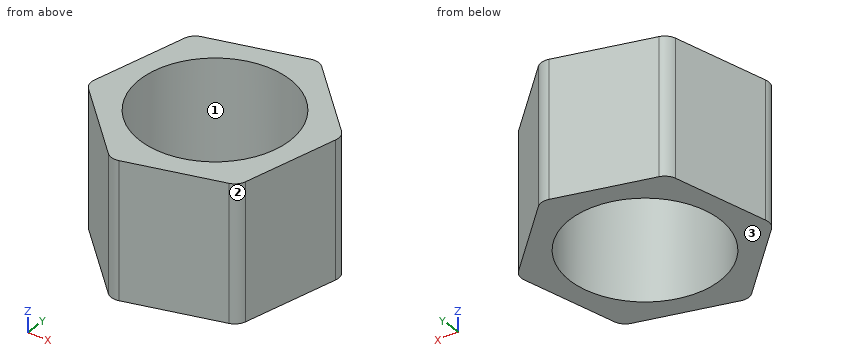
from build123d import *

# Parameters (mm, degrees)
SKETCH3_R           = 11
BOSS_EXTRUDE1_DEPTH = 20
FILLET1_R           = 2


with BuildPart() as part:
    # Sketch3 → Boss-Extrude1 (new body)
    with BuildSketch(Plane.XY):
        Polygon((11.666242226, -11.190716048), (15.524565497, 4.50790411), (3.858323271, 15.698620158), (-11.666242226, 11.190716048), (-15.524565497, -4.50790411), (-3.858323271, -15.698620158), align=None)
        Circle(SKETCH3_R, mode=Mode.SUBTRACT)
    extrude(amount=BOSS_EXTRUDE1_DEPTH)

    # Fillet1
    fillet1_edges = [part.edges().sort_by_distance(p)[0] for p in [
        (-3.858323271, -15.698620158, 10),
        (-15.524565497, -4.50790411, 10),
        (-11.666242226, 11.190716048, 10),
        (3.858323271, 15.698620158, 10),
        (15.524565497, 4.50790411, 10),
        (11.666242226, -11.190716048, 10),
    ]]
    fillet(fillet1_edges, radius=FILLET1_R)


solid = part.part
The listing builds one solid part. Answer for the finished solid, in the listing's coordinates (mm). Face numbers are marked on the shaded views. Give positions to 0.01 mm unless a question says otherwise; leave off trailing zeros. Loops run counter-clockwise (first coordinate to the right, second up) from the corner with the lowest first, then second, coordinate; pieces in that order, holes last. Notation, with made-up numbers: (64, -21) - (121, -21) arc R24 cw to (121, 1) - close; hole circle Ø7 at (64, 22.5). An arc over 180 degrees is marked (long way). Answer as a JSON object with one key per item and string values.
1. A cutting plane is placed at C-C (x = -8). Write down the section's boundary in (y, z), then the cut area to 3 significant figures.
Determined:
{"outline": "(-11.73, 0) - (-7.55, 0) - (-7.55, 20) - (-11.73, 20) - close; (7.55, 0) - (12.26, 0) - (12.26, 20) - (7.55, 20) - close", "area": "178 mm²"}
2. A cutting plane is placed at B-B (y = 0). Write down the section's boundary in (x, z).
Determined:
{"outline": "(-14.42, 0) - (-11, 0) - (-11, 20) - (-14.42, 20) - close; (11, 0) - (14.42, 0) - (14.42, 20) - (11, 20) - close"}
3. For a pull along Y with two mould halves and no side action, classify the marked faces 1, 2 and 3 as pulls with the +Y half, pulls with the -Y half, needs draft (parallel to the pull), parting line crosses it, or undercut.
Determined:
{"face 1": "undercut", "face 2": "pulls with the -Y half", "face 3": "needs draft"}
4. A cutting plane is placed at D-D (y = 13). Write down the section's boundary in (x, z), then the cut area to 3 significant figures.
Determined:
{"outline": "(-5.44, 0) - (6.67, 0) - (6.67, 20) - (-5.44, 20) - close", "area": "242 mm²"}
5. A cutting plane is placed at A-A (z = 2.25). Write down the section's boundary in (x, y), then the cut area to 3 significant figures.
Determined:
{"outline": "(-15.25, -3.39) arc R2 ccw to (-14.69, -5.31) - (-4.69, -14.9) arc R2 ccw to (-2.75, -15.38) - (10.56, -11.51) arc R2 ccw to (11.94, -10.07) - (15.25, 3.39) arc R2 ccw to (14.69, 5.31) - (4.69, 14.9) arc R2 ccw to (2.75, 15.38) - (-10.56, 11.51) arc R2 ccw to (-11.94, 10.07) - close; hole circle Ø22 at (0, 0)", "area": "298 mm²"}
6. Find the intervals of material crossed by L1, parallel to Y at x = 0, z = 10.5; L2, parallel to Y at x = -2, z = 4.25; L3, parallel to X at y = -4.5, z = 2.75, in increasing order. Write a range as [from, to].
Determined:
{"L1": "[-14.58, -11], [11, 14.58]", "L2": "[-15.16, -10.82], [10.82, 14]", "L3": "[-15.2, -10.04], [10.04, 13.31]"}
7. Flat-ended cylindrical pins translate along their axes: pin 1 Ø5 at (x, z) = (6, 15.5) entering from -Y; pin 2 Ø3 at (x, z) = (-8, 13.5) entering from +Y; pin 3 Ø6 at (x, z) = (8.5, 17) entering from +Y. Find the tip coordinate at first contact, or state that the pin passes through.
Determined:
{"pin 1": "y = -13.56", "pin 2": "y = 12.69", "pin 3": "y = 14.12"}
